Here's how the part is built. I have some questions about the finished solid (model axes, mm). Coordinates: 2 decimals unless noted, no trailing zeros. Write each loop counter-clockwise with the first axis right and the second up, starting at its lowest first coordinate (ties: lowest second). Pieces come first, ordered by that corner, then holes.
Item 1: I want a section at C-C (y = 4). Please give me the cut outline in (x, z).
Item 2: Please list where these lines run through material, in increasing order: line 1 (Z direction, x = 0, y = -8.5); line 2 (Z direction, x = 2, y = -10.5); line 3 (Y direction, x = 69, z = -11).
Item 3: I want a section at B-B (x = 60). Please give me the cut outline in (y, z), and give its area (3 significant figures).
Item 4: I'm going to push flat-ended pins straight in: P1, Ø6, axis at x = 63.5, y = 5, coming from the +Z side; P2, Ø8, axis at y = 10.5, z = 23.5, coming from the +X side; P3, Ø6, axis at y = 15, z = -10, coming from the +X side; P4, Ø5, axis at x = 66, y = 1.5, coming from the +Z side. Where does each tip first touch, or does it pass through?
Item 5: I want a section at A-A (y = -21). Please give me the cut outline in (x, z).
Item 6: If we mould it in two halves opening along X, with no side actions, what happens to faces 1 (the face through (50, -14, 0)), 2 (the face through (35.35, -12.325, 23.143)), 3 (the face through (12, 25, -12))? For each: pulls with the +X half, pulls with the -X half, needs draft (parallel to the pull), parting line crosses it, or undercut.
Item 7: I want a section at D-D (z = -2). Count the separate pieces of the cut face and the enclosed holes in it, and give its area (3 significant figures).
from build123d import *

# Parameters (mm, degrees)
F0_R     = 12.5
F0_R_2   = 10
F1_DEPTH = 25
F2_DEPTH = 25
F3_R     = 3
F4_SIZE  = 3


with BuildPart() as f1:
    # F0 (on Front) → F1 (new body)
    with BuildSketch(Plane.XZ):
        with BuildLine():
            ThreePointArc((6.25, -29.341736), (23.318448, -18.874586), (30, 0))
            ThreePointArc((30, 0), (23.318448, 18.874586), (6.25, 29.341736))
            ThreePointArc((6.25, 29.341736), (-30, 0), (6.25, -29.341736))
        make_face()
        Circle(F0_R, mode=Mode.SUBTRACT)
        with BuildLine():
            ThreePointArc((6.25, 29.341736), (23.318448, 18.874586), (30, 0))
            ThreePointArc((30, 0), (23.318448, -18.874586), (6.25, -29.341736))
            Line((6.25, -29.341736), (63.645833, -17.116013))
            ThreePointArc((63.645833, -17.116013), (42.5, 0), (63.645833, 17.116013))
            Line((63.645833, 17.116013), (6.25, 29.341736))
        make_face()
        with BuildLine():
            ThreePointArc((77.5, 0), (73.602428, 11.010175), (63.645833, 17.116013))
            ThreePointArc((63.645833, 17.116013), (42.5, 0), (63.645833, -17.116013))
            ThreePointArc((63.645833, -17.116013), (73.602428, -11.010175), (77.5, 0))
        make_face()
        with Locations((60, 0)):
            Circle(F0_R_2, mode=Mode.SUBTRACT)
    extrude(amount=F1_DEPTH)

    # F0 (on Front) → F2 (join)
    with BuildSketch(Plane.XZ):
        with BuildLine():
            ThreePointArc((6.25, -29.341736), (23.318448, -18.874586), (30, 0))
            ThreePointArc((30, 0), (23.318448, 18.874586), (6.25, 29.341736))
            ThreePointArc((6.25, 29.341736), (-30, 0), (6.25, -29.341736))
        make_face()
        Circle(F0_R, mode=Mode.SUBTRACT)
    extrude(amount=-F2_DEPTH)

    # F3
    f3_edges = [f1.edges().sort_by_distance(p)[0] for p in [
        (-6.25, 25, 29.341736),
    ]]
    fillet(f3_edges, radius=F3_R)

    # F4
    f4_edges = [f1.edges().sort_by_distance(p)[0] for p in [
        (-12.5, 25, 0),
        (50, 0, 0),
    ]]
    chamfer(f4_edges, length=F4_SIZE)


solid = f1.part
Answer:
1. outline: (6.25, -29.34) arc R30 ccw to (30, 0) arc R30 ccw to (6.25, 29.34) arc R30 ccw (long way) to start; hole circle Ø25 at (0, 0)
2. line 1: z = -30 to -12.5, 12.5 to 30
2. line 2: z = -29.93 to -12.34, 12.34 to 29.93
2. line 3: y = -25 to 0
3. outline: (-25, -17.89) - (0, -17.89) - (0, -13) - (-3, -10) - (-25, -10) - close; (-25, 10) - (-3, 10) - (0, 13) - (0, 17.89) - (-25, 17.89) - close
3. area: 386 mm2
4. P1: passes through
4. P2: stops at x = 22.8
4. P3: stops at x = 29.17
4. P4: stops at z = 17.04
5. outline: (6.25, -29.34) - (63.65, -17.12) arc R17.5 ccw to (63.65, 17.12) - (6.25, 29.34) arc R30 ccw (long way) to start; hole circle Ø25 at (0, 0); hole circle Ø20 at (60, 0)
6. face 1: undercut
6. face 2: pulls with the +X half
6. face 3: needs draft
7. separate pieces: 3
7. enclosed holes: 0
7. area: 2,430 mm2
